Can you work these out from the model? Positions are in its coordinate system, mm. Face numbers are marked on the shaded views. A direction names the side the tool comes from. Coordinates: 2 decimals unless noted, no trailing zeros. Loops run counter-clockwise (first coordinate to the right, second up) from the corner with the lowest first, then second, coordinate; pieces in that order, holes last. Notation, with made-up numbers: M -16.5,34 L 4.5,34 A24 cw 4.5,55 Z; hole C 4,53.25 d10. An arc over 180 degrees is marked long. Answer as a JSON object with one key per item and string values. Group by question number.
Item 1: Which directions (+Z, -Z, +X, -X, +Y, -Y) give clear straight access to the entire face, cutting with the end or side of a thin tool? Please do the marked faces 5 and 6.
Item 2: Suppose I cut it at B-B (z = 0). Write out the boundary of the cut face in (x, y) (3 decimals), then the cut area to 3 significant figures.
Item 3: Suppose I cut it at C-C (x = 27). Write out the boundary of the cut face in (y, z).
Item 4: If I drill on line 1 (Y direction, x = 11, z = 0); line 2 (X direction, y = 14, z = -92); line 3 (X direction, y = 43, z = -85), over which ranges is the centre line in solid material (lowest first)?
Item 5: Suppose I cut it at A-A (y = -88.9). Write out the boundary of the cut face in (x, z).
Item 6: I'm going to push flat-ended pins straight in: pin 1 Ø1 at (y, z) = (75, -24) entering from +X; pin 2 Ø4 at (x, z) = (71.5, 17.5) entering from -Y; pin 3 Ø5 at (x, z) = (85.5, 35) entering from -Y. Where does each tip first touch, or does it pass through?
Item 7: Suppose I cut it at D-D (z = -51.5). Write out the boundary of the cut face in (x, y).
Item 8: We'd pull the mould along Y, two halves only. Please class the marked faces 1, 2, 3 and 4: +Y half, -Y half, draft (parallel to the pull), parting line (faces both ways), or undercut.
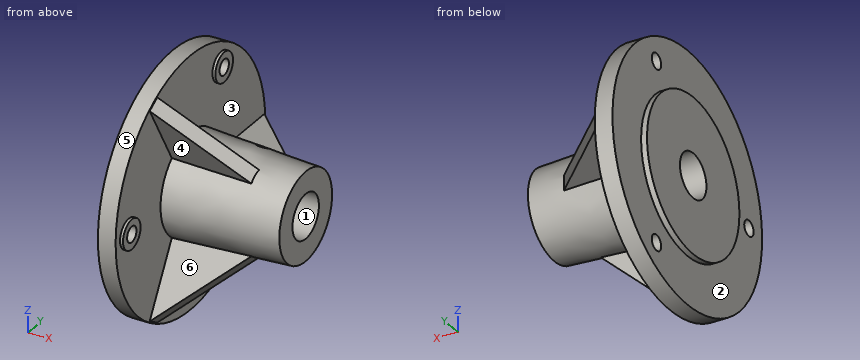
```python
from build123d import *

# Parameters (mm, degrees)
RIB3_REACH              = 192.712
SKETCH5_WALL_W          = 478.079852118
SKETCH5_WALL_H          = 12.7
CIRPATTERN1_COUNT       = 3
SKETCH6_R               = 12.7
BOSS_EXTRUDE1_DEPTH     = 2.54
F_1_2_CLEARANCE_HOLE1_D = 13.49248
SKETCH14_R              = 19.07667
CUT_EXTRUDE1_DEPTH      = 194.798837458


with BuildPart() as part:
    # Sketch2 → Revolve2 (revolve)
    with BuildSketch(Plane.XY, mode=Mode.PRIVATE) as revolve2_sk:
        Polygon((0, 107.95), (0, 66.675), (-5.08, 66.675), (-5.08, 0), (114.3, 0), (114.3, 38.1), (15.24, 43.18), (15.24, 107.95), align=None)
    revolve(revolve2_sk.sketch.rotate(Axis((-82.761666667, 0, 0), (1, 0, 0)), 90), axis=Axis((-82.761666667, 0, 0), (1, 0, 0)))

    # Sketch5 wall → Rib3 (add, up to next)
    with BuildSketch(Plane(origin=(48.706216216, 73.213783784, 0), x_dir=(0.707106781187, -0.707106781187, 0), z_dir=(0.707106781187, 0.707106781187, 0)), mode=Mode.PRIVATE) as rib3_sk1:
        Rectangle(SKETCH5_WALL_W, SKETCH5_WALL_H)
    rib3_tool1 = extrude(rib3_sk1.sketch, amount=-RIB3_REACH, mode=Mode.PRIVATE) - part.part
    rib3 = rib3_tool1.solids().sort_by_distance((48.706216216, 73.213783784, 0))[0]
    add(rib3)

    # CirPattern1: Rib3 ×3 about axis
    cirpattern1_axis = Axis((0, 0, 0), (1, 0, 0))
    for i in range(1, CIRPATTERN1_COUNT):
        add(rib3.rotate(cirpattern1_axis, i * 360 / CIRPATTERN1_COUNT))

    # Sketch6 → Boss-Extrude1 (add)
    with BuildSketch(Plane(origin=(15.24, 0, 0), x_dir=(0, 0, -1), z_dir=(1, 0, 0))):
        with Locations(Location((76.989658396, 44.45, 0), (0, 0, 180))):
            Circle(SKETCH6_R)
        with Locations(Location((0, -88.9, 0), (0, 0, 180))):
            Circle(SKETCH6_R)
        with Locations(Location((-76.989658396, 44.45, 0), (0, 0, 180))):
            Circle(SKETCH6_R)
    extrude(amount=BOSS_EXTRUDE1_DEPTH)

    # 1/2 Clearance Hole1 (through all)
    with Locations(Plane(origin=(17.78, 0, 0), x_dir=(0, 0, -1), z_dir=(1, 0, 0))):
        with Locations((-76.989658396, 44.45), (76.989658396, 44.45), (0, -88.9)):
            Hole(F_1_2_CLEARANCE_HOLE1_D / 2)

    # Sketch13 → 1/8 NPT Tapped Hole1 (revolve, cut)
    with BuildSketch(Plane(origin=(65.257621207, 20.307496892, 35.173616392), x_dir=(0.7626361853665489, -0.5786990925818297, 0.28895226078805086), z_dir=(0.6447969431921082, 0.6447969431921082, -0.41045560551687754))):
        Polygon((0, 0), (0, 39.053866233), (1.5875, 38.1), (1.5875, 6.9342), (4.936185566, 6.9342), (5.1438048, 0), align=None)
    revolve(axis=Axis((65.582834882, 23.478330224, 40.665660824), (-0.05121475197315849, -0.4993438317382925, -0.8648888870168513)), mode=Mode.SUBTRACT)

    # Sketch14 → Cut-Extrude1 (cut, through all)
    with BuildSketch(Plane(origin=(114.3, 0, 0), x_dir=(0, 0, -1), z_dir=(1, 0, 0))):
        Circle(SKETCH14_R)
    extrude(amount=-CUT_EXTRUDE1_DEPTH, mode=Mode.SUBTRACT)


solid = part.part
```
From the geometry:
{
 "1": {"face 5": "+X, -X", "face 6": "+X, -Y"},
 "2": {"outline": "M -5.08,-66.675 L 0,-66.675 L 0,-82.154 L 17.78,-82.154 L 17.78,-76.2 L 15.24,-76.2 L 15.24,-43.18 L 114.3,-38.1 L 114.3,-19.077 L -5.08,-19.077 Z; M -5.08,19.077 L 114.3,19.077 L 114.3,38.1 L 82.172,39.748 L 15.24,106.68 L 15.24,107.95 L 0,107.95 L 0,66.675 L -5.08,66.675 Z; M 0,-107.95 L 15.24,-107.95 L 15.24,-101.6 L 17.78,-101.6 L 17.78,-95.646 L 0,-95.646 Z", "area": "9,410 mm2"},
 "3": {"outline": "M -52.96,-79.03 L -41.96,-85.38 L -15.55,-39.64 A42.58 ccw 42.1,-6.35 L 94.92,-6.35 L 94.92,6.35 L 42.1,6.35 A42.58 ccw -15.55,39.64 L -41.96,85.38 L -52.96,79.03 L -26.55,33.29 A42.58 ccw -26.55,-33.29 Z; hole C 0,0 d38.15"},
 "4": {"line 1": "-107.95 to -95.65, -82.15 to -19.08, 19.08 to 107.95", "line 2": "0 to 15.24", "line 3": "0 to 17.78"},
 "5": {"outline": "M 0,-61.24 L 15.24,-61.24 L 15.24,-12.7 L 17.78,-12.7 L 17.78,-6.75 L 0,-6.75 Z; M 0,6.75 L 17.78,6.75 L 17.78,12.7 L 15.24,12.7 L 15.24,61.24 L 0,61.24 Z"},
 "6": {"pin 1": "x = 15.24", "pin 2": "y = -37.2", "pin 3": "y = -22.59"},
 "7": {"outline": "M -5.08,-42.35 L 0,-42.35 L 0,-94.87 L 15.24,-94.87 L 15.24,-37.07 L 58.79,-37.07 L 66.12,-22.4 L 15.24,-22.4 L 15.24,94.87 L 0,94.87 L 0,42.35 L -5.08,42.35 Z"},
 "8": {"face 1": "undercut", "face 2": "draft", "face 3": "undercut", "face 4": "-Y half"}
}
